from build123d import *

# Parameters (mm, degrees)
F2_DEPTH = 1.6
F3_R     = 0.5


with BuildPart() as f2:
    # F1 (on Top) → F2 (new body)
    with BuildSketch(Plane.XY):
        with BuildLine():
            ThreePointArc((3.15, 6.806431), (0, -7.5), (-3.15, 6.806431))
            ThreePointArc((-3.15, 6.806431), (-0.712379, 13.444051), (-7.35, 15.881672))
            ThreePointArc((-7.35, 15.881672), (-7.403636, 13.003641), (-5.108611, 14.74111))
            ThreePointArc((-5.108611, 14.74111), (-1.915048, 12.00594), (-3.822, 8.258469))
            ThreePointArc((-3.822, 8.258469), (0, -9.1), (3.822, 8.258469))
            ThreePointArc((3.822, 8.258469), (1.915048, 12.00594), (5.108611, 14.74111))
            ThreePointArc((5.108611, 14.74111), (7.403636, 13.003641), (7.35, 15.881672))
            ThreePointArc((7.35, 15.881672), (0.712379, 13.444051), (3.15, 6.806431))
        make_face()
    extrude(amount=F2_DEPTH)

    # F3
    f3_edges = [f2.edges().sort_by_distance(p)[0] for p in [
        (5.108611, 14.74111, 0.8),
        (-5.108611, 14.74111, 0.8),
    ]]
    fillet(f3_edges, radius=F3_R)


solid = f2.part
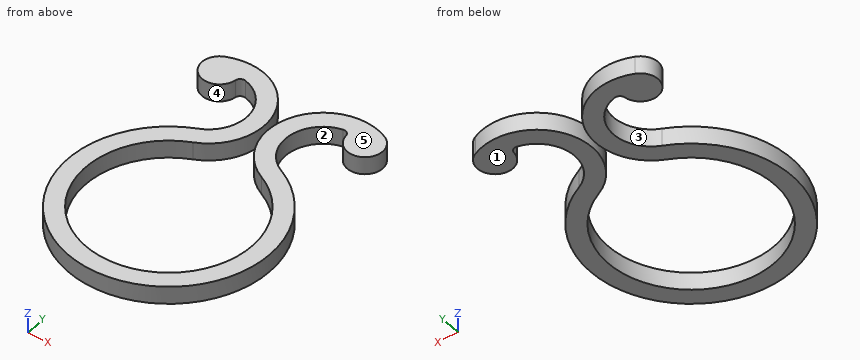
Design review of the part built by this model. Coordinates are the model's own, in mm. Face numbers are marked on the shaded views. A direction names the side the tool comes from. Give positions to 0.01 mm unless a question says otherwise; leave off trailing zeros. Loops run counter-clockwise (first coordinate to the right, second up) from the corner with the lowest first, then second, coordinate; pieces in that order, holes last. Notation, with made-up numbers: M -28.75,85.5 L 3.25,85.5 A8 cw 3.25,89.5 Z; hole C -33,-16.5 d5. An arc over 180 degrees is marked long. Write item = value, one per line.
Q1. To check wall thickness, follow line 1 (X direction, y = 13.5, z = 1.45); line 2 (Y direction, x = 5.75, z = 0.3); line 3 (X direction, y = 0, z = 0.5). State the ranges of each line that lie inside material, in increasing order. Write a range as [from, to].
Output values:
line_1 = [-7.98, -5.38], [-2.62, -0.74], [0.74, 2.62], [5.38, 7.98]
line_2 = [-7.05, -4.82], [4.82, 7.05], [13.13, 16.32]
line_3 = [-9.1, -7.5], [7.5, 9.1]
Q2. Insertion check: pin 1 (10 mm diameter, centred on x = 2.5, y = 7, fed in from +Z). The pin has a flat end and moves straight along its axis. Give the tip position at first contact, or say it passes through.
Output values:
pin_1 = 1.6
Q3. We need section B-B (x = -2.5). Give the boundary of the cut face in (y, z).
Output values:
outline = M -8.75,0 L -7.07,0 L -7.07,1.6 L -8.75,1.6 Z; M 7.17,0 L 9.34,0 L 9.34,1.6 L 7.17,1.6 Z; M 13.34,0 L 15.52,0 L 15.52,1.6 L 13.34,1.6 Z
Q4. We need section A-A (y = -3.5). Give the boundary of the cut face in (x, z), plus the area to 3 significant figures.
Output values:
outline = M -8.4,0 L -6.63,0 L -6.63,1.6 L -8.4,1.6 Z; M 6.63,0 L 8.4,0 L 8.4,1.6 L 6.63,1.6 Z
area = 5.65 mm^2
Q5. Draft analysis for pull direction Y (two halves, no side actions). For the marked faces 3, 4 and 5, state which applies: +Y half, -Y half, draft (parallel to the pull), parting line (faces both ways), or undercut.
Output values:
face_3 = undercut
face_4 = undercut
face_5 = draft
Q6. For the marked faces 1 and 2, list the 3-axis set-ups (+Z, -Z, +X, -X, +Y, -Y) from which the entire face can be reached by the end or side of a thin tool; tool diameter is ignored.
Output values:
face_1 = -Z, +X, -X, +Y, -Y
face_2 = +Z, -Z
Q7. We need section C-C (y = 0). Give the boundary of the cut face in (x, z).
Output values:
outline = M -9.1,0 L -7.5,0 L -7.5,1.6 L -9.1,1.6 Z; M 7.5,0 L 9.1,0 L 9.1,1.6 L 7.5,1.6 Z
